Input: dimensioned drawing with shaded views. Units: mm. Origin: part minimum x, y, z. Round coordinates to 2 decimals unless told otherwise and drop trailing zeros. Order: outer loops, then holes, each group sorted by start corner. A loop starts at its lowest first (then second) coordinate and runs counter-clockwise, first axis right, second up. Notation, with made-up numbers: (2, 33.5) - (40, 33.5) arc R26 cw to (40, 54.5) - close; hole circle Ø5 at (-26.5, -40). An arc over 180 degrees is marked (long way). Put each result on its own line as item: value. Start each with the question number.
(1) Material intervals for L1, parallel to X at y = 87.45, z = 1.15; L2, parallel to X at y = 87, z = 0.1, sorted ascending. Write a range as [from, to].
(2) Pin query (flat end, axial travel): P1, Ø4, axis at x = 46.5, y = 47.5, coming from the -Z side. Return the tip coordinate at first contact, or that it passes through.
(3) Section A-A (z = 1.6). Output: boundary loops of the cut face in (x, y), and give its area (3 significant figures).
(4) Section B-B (x = 17.45). Output: boundary loops of the cut face in (y, z).
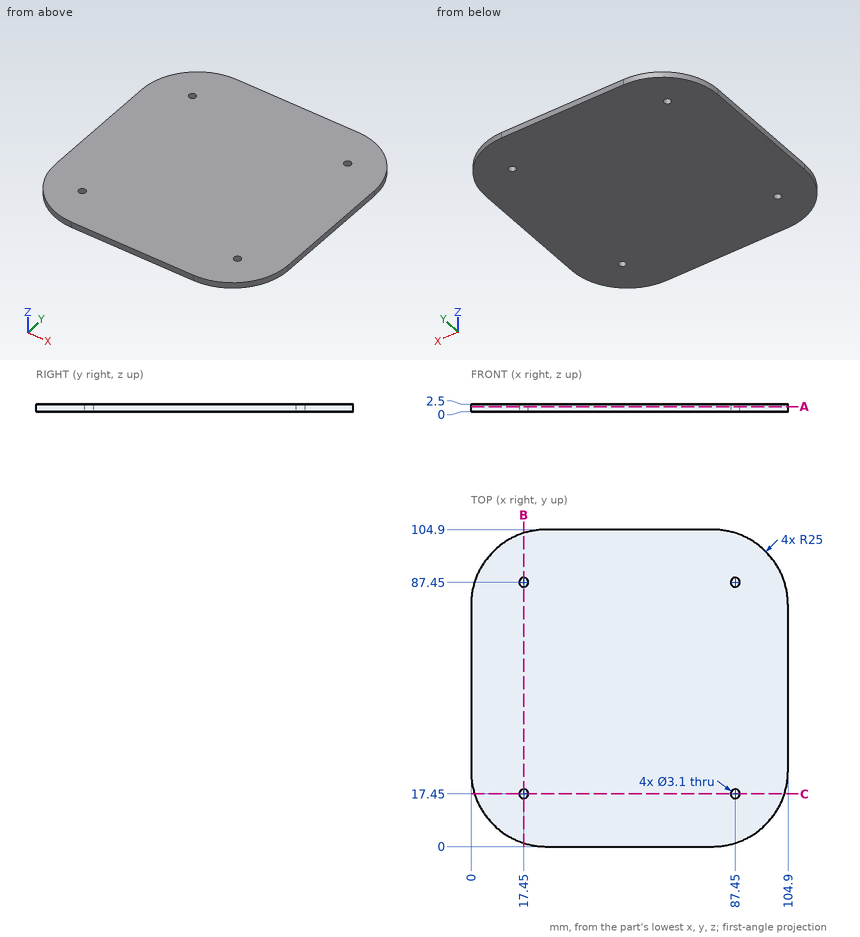
Checks:
1. L1: x = [1.17, 15.9], [19, 85.9], [89, 103.73]
1. L2: x = [1.03, 15.97], [18.93, 85.97], [88.93, 103.87]
2. P1: stops at z = 0
3. outline: (0, 25) arc R25 ccw to (25, 0) - (79.9, 0) arc R25 ccw to (104.9, 25) - (104.9, 79.9) arc R25 ccw to (79.9, 104.9) - (25, 104.9) arc R25 ccw to (0, 79.9) - close; hole circle Ø3.1 at (17.45, 17.45); hole circle Ø3.1 at (17.45, 87.45); hole circle Ø3.1 at (87.45, 17.45); hole circle Ø3.1 at (87.45, 87.45)
3. area: 10,400 mm²
4. outline: (1.17, 0) - (15.9, 0) - (15.9, 2.5) - (1.17, 2.5) - close; (19, 0) - (85.9, 0) - (85.9, 2.5) - (19, 2.5) - close; (89, 0) - (103.73, 0) - (103.73, 2.5) - (89, 2.5) - close
